Solid Edge part; units mm, degrees
sketch "Sketch1" plane through (0, 0, 0) normal (0, -1, 0) x (1, 0, 0)
  line L0 (-6.65, 9.9) -> (6.65, 9.9)
  line L1 (6.65, 9.9) -> (6.65, 16.1)
  line L2 (6.65, 16.1) -> (-6.65, 16.1)
  line L3 (-6.65, 16.1) -> (-6.65, 9.9)
  line L4 (9, 10.2836) -> (9, 17)
  arc A0 (9, 17) -> (7, 19) centre (7, 17) ccw
  line L5 (7, 19) -> (-7, 19)
  arc A1 (-7, 19) -> (-9, 17) centre (-7, 17) ccw
  line L6 (-9, 17) -> (-9, 10.2836)
  arc A2 (-9, 10.2836) -> (-8.7878, 8.4533) centre (-1, 10.2836) ccw
  line L7 (-6.7122, -0.3777) -> (-8.7878, 8.4533)
  arc A3 (-6.5, -2.2081) -> (-6.7122, -0.3777) centre (-14.5, -2.2081) ccw
  line L8 (-6.5, -15.1458) -> (-6.5, -2.2081)
  line L9 (-4, -15.1458) -> (-6.5, -15.1458)
  line L10 (-4, -15.1458) -> (-4, -1.2806)
  line L11 (4, -15.1458) -> (4, -1.2806)
  line L12 (4, -15.1458) -> (6.5, -15.1458)
  line L13 (6.5, -15.1458) -> (6.5, -2.2081)
  arc A4 (6.5, -2.2081) -> (6.7122, -0.3777) centre (14.5, -2.2081) cw
  line L14 (6.7122, -0.3777) -> (8.7878, 8.4533)
  arc A5 (9, 10.2836) -> (8.7878, 8.4533) centre (1, 10.2836) cw
  arc A6 (-4, -1.2806) -> (4, -1.2806) centre (0, 0) cw
  dimension "D1" = 6.65
  dimension "D2" = 6.65
extrude "Protrusion1" add sketch "Sketch1" against normal blind 10
sketch "Sketch2" plane through (6.5, 6, -9.599) normal (1, 0, 0) x (0, 0, 1)
  circle A0 centre (-0.5467, 1) radius 1.5773
  dimension "D1" = 0.5467
extrude "Cutout1" cut sketch "Sketch2" against normal up to vertex (13 mm away)
sketch "Sketch3" plane through (-6.5, 6, -9.599) normal (-1, 0, 0) x (0, 0, -1)
  line L0 (-1.1853, 4) -> (-2.9174, 1)
  line L1 (-2.9174, 1) -> (-1.1853, -2)
  line L2 (-1.1853, -2) -> (2.2788, -2)
  line L3 (2.2788, -2) -> (4.0108, 1)
  line L4 (4.0108, 1) -> (2.2788, 4)
  line L5 (2.2788, 4) -> (-1.1853, 4)
extrude "ExtrudedCutout_2" cut sketch "Sketch3" against normal blind 1
fillet "Round_1" radius 4 4 edges at (-5.25, 0, -15.1458) (-5.25, 10, -15.1458) (5.25, 10, -15.1458) (5.25, 0, -15.1458)
sketch "Sketch4" plane through (0, 10, 4.4271) normal (0, 1, 0) x (-1, 0, 0)
  line L0 (-10, 7.0729) -> (10, 7.0729)
  line L1 (10, 7.0729) -> (10, 10.0729)
  line L2 (10, 10.0729) -> (-10, 10.0729)
  line L3 (-10, 10.0729) -> (-10, 7.0729)
extrude "ExtrudedCutout_3" cut sketch "Sketch4" against normal blind 5
fillet "Round_5" radius 1 4 edges at (7.825, 10, 11.5) (7.825, 10, 14.5) (-7.825, 10, 11.5) (-7.825, 10, 14.5)
The model under review builds one solid part; all positions refer to its coordinate system, in mm. A direction names the side the tool comes from. Round coordinates to 2 decimals unless told otherwise and drop trailing zeros. Loops run counter-clockwise (first coordinate to the right, second up) from the corner with the lowest first, then second, coordinate; pieces in that order, holes last. Notation, with made-up numbers: (-13.5, 14.5) - (4.5, 14.5) arc R11 cw to (4.5, 33.5) - close; hole circle Ø11 at (44.5, 87). An arc over 180 degrees is marked (long way). Use a Markdown table: item, result. Add a question column.
Q1. The part is to be moulded in two halves that separate along X. For faces 1 (the face through (-8, 5, 13)), 2 (the face through (0, 5, 16.1)), 3 (the face through (-8.95, 4.93, 9.38)), say which applies: pulls with the +X half, pulls with the -X half, needs draft (parallel to the pull), parting line crosses it, or undercut.
Q2. Add section D-D (x = -7.5). State the section outline as (y, z) points.
Q3. Machinability: for faces 4 (the face through (-8, 7, 14.5)), 5 (the face through (-6.65, 4, 13)), 6 (the face through (-6.007, 6.479, -7.536)), which of the approach directions +Z, -Z, +X, -X, +Y, -Y give a long, thin tool a straight path to every point of the face, cutting with its end or side? Answer none if there is none.
Q4. Add section A-A (x = 0). State the section outline as (y, z) points.
Q5. Insertion check: pin 1 Ø2.5 at (x, y) = (-8.5, 8) entering from +Z; pin 2 Ø2.5 at (x, z) = (-7.5, 13.5) entering from +Y; pin 3 Ø5 at (y, z) = (3, -5.5) entering from +X; pin 4 Ø1.9 at (y, z) = (5, -10.15) entering from +X. Each pin has a flat end and moves straight along its axis. Give the tip position at first contact, or say it passes through.
Q6. Add section B-B (z = 13). State the section outline as (x, y) points.
Q7. Add section C-C (y = 1.25). State the section outline as (x, z) points, plus the area to 3 significant figures.
Q8. For probe 1 along Z at (x, y) = (-4.95, 5); probe 2 along X at (y, z) = (2.75, -6); probe 3 along Z at (x, y) = (-2, 9.25), list the stretches that pass through material, from the lowest coordinate up.
Worked answers:
| question | item | result |
|---|---|---|
| 1 | face 1 | needs draft |
| 1 | face 2 | undercut |
| 1 | face 3 | pulls with the -X half |
| 2 | outline | (0, 2.97) - (10, 2.97) - (10, 10.5) arc R1 ccw to (9, 11.5) - (5, 11.5) - (5, 14.5) - (9, 14.5) arc R1 ccw to (10, 15.5) - (10, 18.94) - (0, 18.94) - close |
| 3 | face 4 | +X, -X, +Y |
| 3 | face 5 | +Y, -Y |
| 3 | face 6 | -X |
| 4 | outline | (0, 4.2) - (10, 4.2) - (10, 9.9) - (0, 9.9) - close; (0, 16.1) - (10, 16.1) - (10, 19) - (0, 19) - close |
| 5 | pin 1 | z = 18.98 |
| 5 | pin 2 | y = 9.66 |
| 5 | pin 3 | x = 6.5 |
| 5 | pin 4 | through |
| 6 | outline | (-9, 0) - (-6.65, 0) - (-6.65, 5) - (-9, 5) - close; (6.65, 0) - (9, 0) - (9, 5) - (6.65, 5) - close |
| 7 | outline | (-9, 10.28) arc R8 ccw to (-8.79, 8.45) - (-6.71, -0.38) arc R8 cw to (-6.5, -2.21) - (-6.5, -14.05) - (-4, -14.05) - (-4, -1.28) arc R4.2 cw (long way) to (4, -1.28) - (4, -14.05) - (6.5, -14.05) - (6.5, -2.21) arc R8 cw to (6.71, -0.38) - (8.79, 8.45) arc R8 ccw to (9, 10.28) - (9, 17) arc R2 ccw to (7, 19) - (-7, 19) arc R2 ccw to (-9, 17) - close; hole (-6.65, 9.9) - (6.65, 9.9) - (6.65, 16.1) - (-6.65, 16.1) - close |
| 7 | area | 280 mm² |
| 8 | probe 1 | -15.15 to -11.72, -8.57 to 9.9, 16.1 to 19 |
| 8 | probe 2 | -6.5 to -4, 4 to 6.5 |
| 8 | probe 3 | 3.69 to 9.9, 16.1 to 19 |
